Autodesk Inventor part; units mm, degrees
ref_plane "Work Plane1" through (15.875, 70.0104, 0) normal (0, -1, 0) x (0, 0, 1)
ref_plane "YZ Plane" through (0, 0, 0) normal (1, 0, 0) x (0, 1, 0)
ref_plane "XZ Plane" through (0, 0, 0) normal (0, 1, 0) x (-1, 0, 0)
sketch "Sketch1" plane through (0, 0, 0) normal (0, 0, 1) x (1, 0, 0)
  line L0 (0, 0) -> (15.875, 0)
  line L1 (15.875, 0) -> (15.875, 77.724)
  line L2 (15.875, 77.724) -> (0, 77.724)
  line L3 (0, 77.724) -> (0, 0)
  dimension "d0" = 77.724
  dimension "d1" = 15.875
extrude "Extrusion1" add sketch "Sketch1" along normal blind 3.175
sketch "Sketch2" plane through (0, 0, 3.175) normal (0, 0, 1) x (1, 0, 0)
  line L0 (0, 0) -> (15.875, 0)
  line L1 (15.875, 77.724) -> (0, 77.724)
  line L2 (3.175, 0) -> (12.7, 0)
  line L3 (12.7, 0) -> (12.7, 3.175)
  line L4 (12.7, 3.175) -> (3.175, 3.175)
  line L5 (3.175, 3.175) -> (3.175, 0)
  line L6 (7.9375, 3.175) -> (7.9375, 0) construction
  line L7 (7.9375, 77.724) -> (7.9375, 0) construction
  dimension "d4" = 9.525
  dimension "d6" = 3.175
extrude "Extrusion2" cut sketch "Sketch2" against normal through all
sketch "Sketch3" plane through (0, 0, 3.175) normal (0, 0, 1) x (1, 0, 0)
  circle A0 centre (7.9375, 77.7875) radius 11.1125
  dimension "d11" = 22.225
extrude "Extrusion3" cut sketch "Sketch3" against normal blind 3.175
ref_plane "Work Plane1" through (15.875, 70.0104, 0) normal (0, -1, 0) x (0, 0, 1)
sketch "Sketch6" plane through (15.875, 70.0104, 0) normal (0, -1, 0) x (0, 0, 1)
  line L0 (3.1705, 0.0025) -> (0, 0.0025) construction
  line L1 (1.5853, 0.0025) -> (1.5853, 15.875) construction
  circle A0 centre (1.5853, 7.9388) radius 0.6177
  point P0 (0, 15.875)
hole "Hole3" at (7.9362, 70.0104, 1.5853) direction (0, -1, 0) diameter 1.7018 depth 33.02 tip angle 118
sketch "Sketch7" plane through (15.875, 0, 0) normal (0, -1, 0) x (1, 0, 0)
  line L0 (-15.875, 0) -> (0, 0) construction
  line L1 (0, 0) -> (0, 3.175) construction
  line L2 (0, 3.175) -> (-15.875, 3.175) construction
  line L3 (-15.875, 3.175) -> (-15.875, 0) construction
  line L4 (-7.9375, 3.175) -> (-7.9375, 0) construction
  circle A0 centre (-14.2875, 1.5875) radius 0.7756
  line L5 (-15.875, 0) -> (-15.875, 3.175) construction
  circle A1 centre (-1.5875, 1.5875) radius 0.7756
  point P0 (-3.175, 3.175)
  dimension "d36" = 15.875
  dimension "d37" = 6.35
hole "Hole4" at (14.2875, 0, 1.5875) at (1.5875, 0, 1.5875) direction (0, 1, 0) diameter 1.7018 depth 25.4 tip angle 118
properties part number "2f1ar" material "Brass, Soft Yellow"
Model file for the job. Use its own axes, mm. A direction names the side the tool comes from. Give positions to 0.01 mm unless a question says otherwise; leave off trailing zeros. Order: outer loops, then holes, each group sorted by start corner. A loop starts at its lowest first (then second) coordinate and runs counter-clockwise, first axis right, second up. Notation, with made-up numbers: (-27, 60) - (-2, 60) arc R22 cw to (-2, 95) - close; hole circle Ø6 at (57.5, 28). An arc over 180 degrees is marked (long way). One line per item, written item: value.
Item 1: Wall check: line 1 (X direction, y = 22.5, z = 1.45) (3 decimals); line 2 (X direction, y = 38, z = 1.45) (3 decimals); line 3 (X direction, y = 10.5, z = 1.9) (3 decimals). Give the ranges that are in metal, low to high.
Response values:
line 1: 0 to 0.748, 2.427 to 13.448, 15.127 to 15.875
line 2: 0 to 7.096, 8.776 to 15.875
line 3: 0 to 0.796, 2.379 to 13.496, 15.079 to 15.875
Item 2: Slice it at A-A (y = 12.5). List the corners of the cut face in (x, z) (1 decimal).
Response values:
outline: (0, 0) - (15.9, 0) - (15.9, 3.2) - (0, 3.2) - close; hole circle Ø1.7 at (1.6, 1.6); hole circle Ø1.7 at (14.3, 1.6)
Item 3: Tool access for faces 5 (the cylindrical face through (7.093, 51.641, 1.475)), 6 (the flat face through (15, 0, 2.3)), 7 (the cylindrical face through (15.12, 12.88, 1.77)), 8 (the flat face through (0, 35, 2)), 9 (the flat face through (12.7, 2, 2)): list every direction of +Z, -Z, +X, -X, +Y, -Y with a clear straight run to the whole face (end or side of a thin tool).
Response values:
face 5: +Y
face 6: +Z, -Z, +X, -X, -Y
face 7: -Y
face 8: +Z, -Z, -X, +Y, -Y
face 9: +Z, -Z, -Y
Item 4: Slice it at B-B (y = 44). List the corners of the cut face in (x, z) (3 decimals).
Response values:
outline: (0, 0) - (15.875, 0) - (15.875, 3.175) - (0, 3.175) - close; hole circle Ø1.702 at (7.936, 1.585)
Item 5: Pin check, flat tips, straight feed: pin 1 Ø1.4 at (x, z) = (14.29, 1.59) entering from +Y; pin 2 Ø1 at (x, z) = (12, 2.5) entering from -Y (3 decimals). Stop position of each tip, or through.
Response values:
pin 1: y = 69.2
pin 2: y = 3.175
Item 6: Two-plate mould, pull along Z, no slides. Class faces 1 (the conical face through (8.1, 36.6, 1.7)), 2 (the flat face through (8, 35, 0)), 3 (the flat face through (2.3, 0, 2.3)), 4 (the cylindrical face through (1.332, 12.878, 0.776)): released by +Z, released by -Z, zero draft, split by the parting line, or undercut.
Response values:
face 1: undercut
face 2: released by -Z
face 3: zero draft
face 4: undercut
Item 7: Slice it at C-C (x = 6.5). List the corners of the cut face in (y, z) (3 decimals).
Response values:
outline: (3.175, 0) - (66.768, 0) - (66.768, 3.175) - (3.175, 3.175) - close
